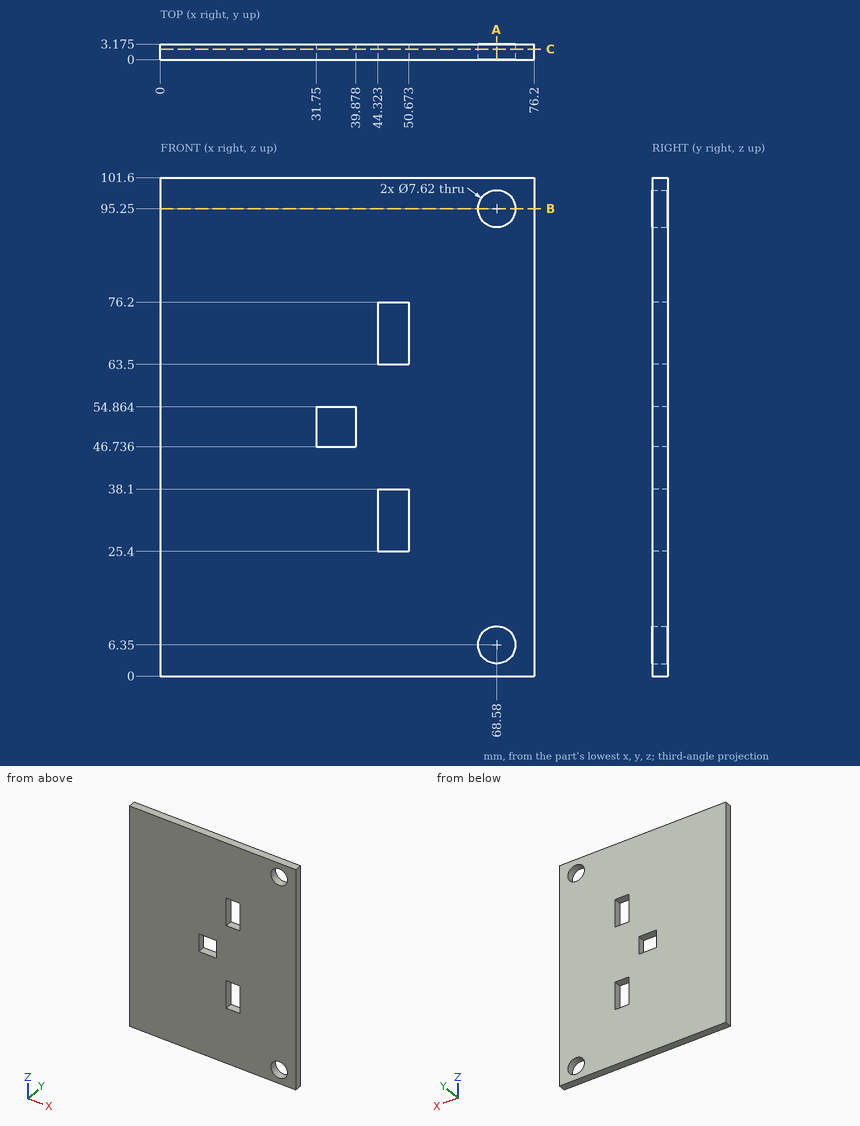
For this review, use the dimensioned drawing (mm, ordinates from the lowest corner) and the shaded views. Give positions to 0.01 mm unless a question says otherwise; leave off trailing zeros. Order: outer loops, then holes, each group sorted by start corner. A loop starts at its lowest first (then second) coordinate and runs counter-clockwise, first axis right, second up. Notation, with made-up numbers: (21, 62) - (62, 62) arc R30 cw to (62, 92) - close; hole circle Ø6 at (54, 71). An arc over 180 degrees is marked (long way). Use CSV: the item, a comma, the result in double quotes. Start each with the question number.
Q1. We need section C-C, the plane y = 2.15. Write out the cut boundary in (x, z).
Q2. We need section A-A, the plane x = 68.58. Write out the cut boundary in (y, z) (3 decimals), and give its area (3 significant figures).
Q3. We need section B-B, the plane z = 95.25. Write out the cut boundary in (x, y) (3 decimals), and give its area (3 significant figures).
Q4. To check wall thickness, follow line 1 along Z through (x, y) = (49, 1.95); line 2 along Z through (x, y) = (68.58, 2.4); line 3 along X through (y, z) = (1.55, 6.35). State the ranges of each line that lie inside material, in increasing order. Write a range as [from, to].
Outcome:
1,outline,"(0, 0) - (76.2, 0) - (76.2, 101.6) - (0, 101.6) - close; hole (31.75, 46.74) - (39.88, 46.74) - (39.88, 54.86) - (31.75, 54.86) - close; hole (44.32, 25.4) - (50.67, 25.4) - (50.67, 38.1) - (44.32, 38.1) - close; hole (44.32, 63.5) - (50.67, 63.5) - (50.67, 76.2) - (44.32, 76.2) - close; hole circle Ø7.62 at (68.58, 6.35); hole circle Ø7.62 at (68.58, 95.25)"
2,outline,"(0, 0) - (3.175, 0) - (3.175, 2.54) - (0, 2.54) - close; (0, 10.16) - (3.175, 10.16) - (3.175, 91.44) - (0, 91.44) - close; (0, 99.06) - (3.175, 99.06) - (3.175, 101.6) - (0, 101.6) - close"
2,area,"274 mm^2"
3,outline,"(0, 0) - (64.77, 0) - (64.77, 3.175) - (0, 3.175) - close; (72.39, 0) - (76.2, 0) - (76.2, 3.175) - (72.39, 3.175) - close"
3,area,"218 mm^2"
4,line 1,"z = [0, 25.4], [38.1, 63.5], [76.2, 101.6]"
4,line 2,"z = [0, 2.54], [10.16, 91.44], [99.06, 101.6]"
4,line 3,"x = [0, 64.77], [72.39, 76.2]"
